Study the drawing (mm; zero at the part's minimum x, y, z) and answer. A direction names the side the tool comes from. Coordinates: 2 decimals unless noted, no trailing zeros. Loops run counter-clockwise (first coordinate to the right, second up) from the corner with the lowest first, then second, coordinate; pieces in that order, holes last. Notation, with made-up numbers: M 4,-18 L 22,-18 A20 cw 22,1 Z; hole C -30,27 d9. An arc over 180 degrees is marked long. Use one line per item in the form item = value. Start each with the question number.
1. Find the intervals of material crossed by probe 1 along X at (y, z) = (2, 2.6); probe 2 along Z at (x, y) = (7.75, 10), in increasing order. Write a range as [from, to].
2. The part is cut by section B-B (z = 1.2). Give the vertices of the cut face in (x, y).
3. For a pull along X with two mould halves and no side action, classify the marked faces 1, 2, 3 and 4 as released by +X, released by -X, zero draft, split by the parting line, or undercut.
4. The part is cut by section A-A (x = 2). Give the vertices of the cut face in (y, z), plus the area to 3 significant figures.
5. A tool of negligible diameter and unlimited length cuts with its end or side. For the marked faces 5 and 6, from which of +Z, -Z, +X, -X, +Y, -Y can it reach the whole face along a straight path? Write none if from no direction.
6. A flat-ended cylindrical pin translates along its axis: pin 1 (5 mm diameter, centred on x = 7, y = 5, fed in from -Z). Find the tip coordinate at first contact, or state that the pin passes through.
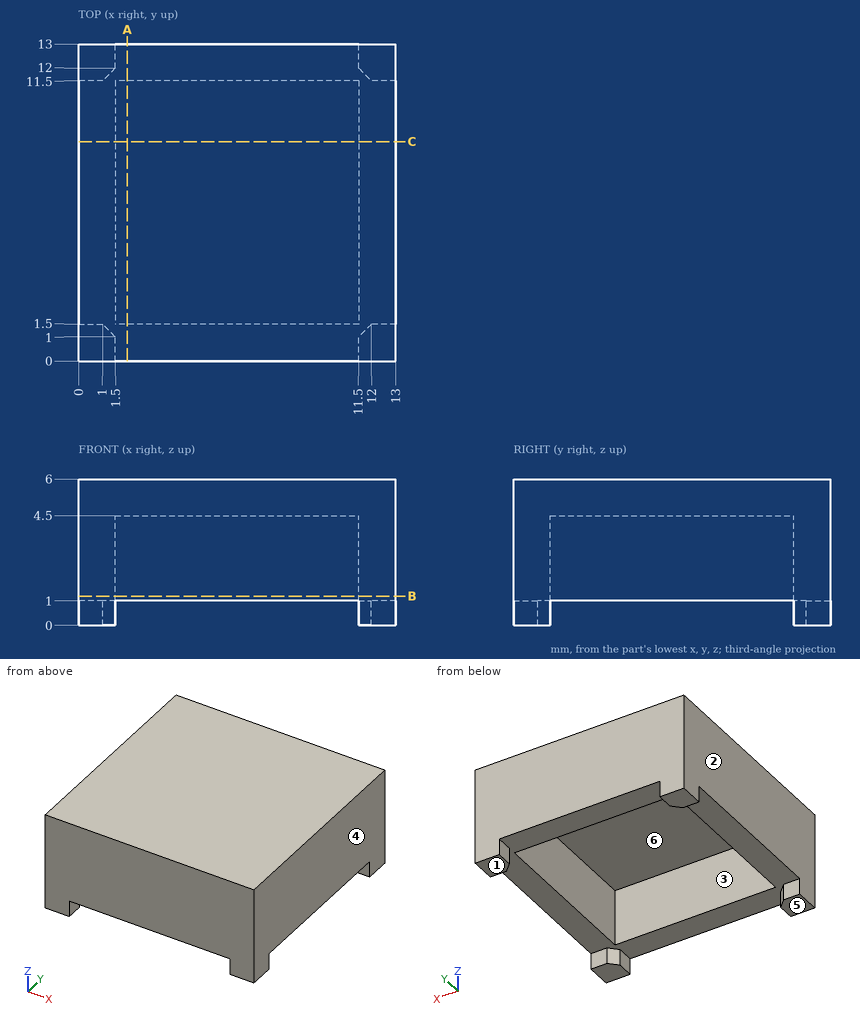
Computed values:
q1.probe_1 = [0, 1.5], [11.5, 13]
q1.probe_2 = [4.5, 6]
q2.outline = M 0,0 L 13,0 L 13,13 L 0,13 Z; hole M 1.5,1.5 L 11.5,1.5 L 11.5,11.5 L 1.5,11.5 Z
q3.face_1 = zero draft
q3.face_2 = released by -X
q3.face_3 = undercut
q3.face_4 = released by +X
q4.outline = M 0,1 L 1.5,1 L 1.5,4.5 L 11.5,4.5 L 11.5,1 L 13,1 L 13,6 L 0,6 Z
q4.area = 30.0 mm²
q5.face_5 = -Z, +X, -X, +Y, -Y
q5.face_6 = -Z
q6.pin_1 = 4.5
